CAD build for the part. Positions are in the model's coordinates, mm. Round coordinates to 2 decimals unless told otherwise and drop trailing zeros. Order: outer loops, then holes, each group sorted by start corner. A loop starts at its lowest first (then second) coordinate and runs counter-clockwise, first axis right, second up.
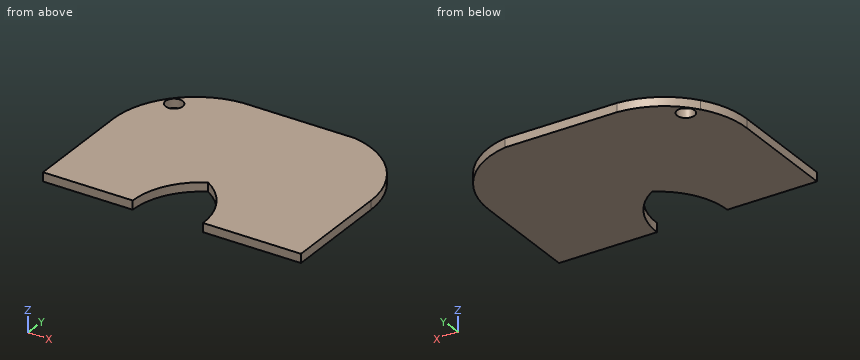
```python
from build123d import *

# Parameters (mm, degrees)
F0_R     = 9.847408
F0_W     = 127.524496
F0_H     = 93.789673
F1_DEPTH = 10.16


with BuildPart() as f1:
    # F0 (on Top) → F1 (new body)
    with BuildSketch(Plane.XY):
        with BuildLine():
            ThreePointArc((-126.299633, 109.920687), (-139.400604, 83.911871), (-143.911943, 55.141368))
            Line((-143.911943, 55.141368), (-56.138069, 55.141368))
            Line((-56.138069, 55.141368), (-56.138069, 148.931041))
            ThreePointArc((-56.138069, 148.931041), (-95.592892, 137.292738), (-126.299633, 109.920687))
        make_face()
        with Locations((-110.678472, 111.924551)):
            Circle(F0_R, mode=Mode.SUBTRACT)
        with BuildLine():
            Line((-56.138069, 55.141368), (-143.911943, 55.141368))
            Line((-143.911943, 55.141368), (-143.911943, -68.781622))
            Line((-143.911943, -68.781622), (-41.689414, -68.781622))
            ThreePointArc((-41.689414, -68.781622), (-30.327603, -28.643107), (0, 0))
            ThreePointArc((0, 0), (28.519495, -29.543531), (38.738407, -69.314823))
            Line((38.738407, -69.314823), (150.395036, -69.314823))
            Line((150.395036, -69.314823), (150.395036, 55.141368))
            Line((150.395036, 55.141368), (71.386427, 55.141368))
            Line((71.386427, 55.141368), (-56.138069, 55.141368))
        make_face()
        with Locations((7.624179, 102.036204)):
            Rectangle(F0_W, F0_H)
        with BuildLine():
            Line((71.386427, 148.931041), (71.386427, 55.141368))
            Line((71.386427, 55.141368), (150.395036, 55.141368))
            ThreePointArc((150.395036, 55.141368), (128.010449, 116.457889), (71.386427, 148.931041))
        make_face()
    extrude(amount=-F1_DEPTH)


solid = f1.part
```
1. Cut at B-B, the plane z = -3. Write the cut outline in (x, y), and give its area (3 significant figures).
2. Cut at A-A, the plane y = -39. Write the cut outline in (x, z).
3. Cut at C-C, the plane x = 103. Write the cut outline in (y, z).
4. Pin check, flat tips, straight feed: P1, Ø3, axis at x = 29, z = -2, coming from the -Y side; P2, Ø17.5, axis at x = -110.68, y = 111.92, coming from the +Z side. Stop position of each tip, or through.
5. Drill centre lines: line 1 (X direction, y = -27, z = -4); line 2 (Y direction, x = -46.5, z = -0.5); line 3 (X direction, y = -0.5, z = -5.5). Where is each one in solid material? Low to high.
Outcome:
1. outline: (-143.91, -68.78) - (-41.69, -68.78) arc R78.47 cw to (0, 0) arc R80.43 cw to (38.74, -69.31) - (150.4, -69.31) - (150.4, 55.14) arc R95.17 ccw to (71.39, 148.93) - (-56.14, 148.93) arc R94 ccw to (-126.3, 109.92) arc R94 ccw to (-143.91, 55.14) - close; hole circle Ø19.69 at (-110.68, 111.92)
1. area: 56,200 mm2
2. outline: (-143.91, -10.16) - (-35.6, -10.16) - (-35.6, 0) - (-143.91, 0) - close; (33.02, -10.16) - (150.4, -10.16) - (150.4, 0) - (33.02, 0) - close
3. outline: (-69.31, -10.16) - (137.45, -10.16) - (137.45, 0) - (-69.31, 0) - close
4. P1: stops at y = -33.32
4. P2: passes through
5. line 1: x = -143.91 to -29.3, 27.04 to 150.4
5. line 2: y = -68.78 to 148.93
5. line 3: x = -143.91 to -0.93, 0.81 to 150.4
